from build123d import *

# Parameters (mm, degrees)
F0_W      = 108
F0_H      = 130
F1_DEPTH  = 70
F2_R      = 6.5
F3_DEPTH  = 70.001
F4_W      = 70
F4_H      = 50
F5_DEPTH  = 25
F6_W      = 108
F6_H      = 82
F7_DEPTH  = 25
F9_DEPTH  = 108.001
F10_R     = 10
F11_DEPTH = 20
F12_R     = 10
F13_DEPTH = 20
F14_W     = 44
F14_H     = 20
F14_W_2   = 20
F14_H_2   = 55
F15_DEPTH = 5


with BuildPart() as f1:
    # F0 (on Right) → F1 (new body)
    with BuildSketch(Plane.YZ):
        Rectangle(F0_W, F0_H)
    extrude(amount=-F1_DEPTH)

    # F2 (on face) → F3 (cut, through all)
    with BuildSketch(Plane(origin=(-70, 0, 0), x_dir=(0, -1, 0), z_dir=(-1, 0, 0))):
        with Locations((-42, 47)):
            Circle(F2_R)
        with Locations((42, 47)):
            Circle(F2_R)
        with Locations((-42, -47)):
            Circle(F2_R)
        with Locations((42, -47)):
            Circle(F2_R)
    extrude(amount=-F3_DEPTH, mode=Mode.SUBTRACT)

    # F4 (on face) → F5 (cut)
    with BuildSketch(Plane(origin=(0, 0, -65), x_dir=(1, 0, 0), z_dir=(0, 0, -1))):
        with Locations((-35, 0)):
            Rectangle(F4_W, F4_H)
    extrude(amount=-F5_DEPTH, mode=Mode.SUBTRACT)

    # F6 (on face) → F7 (cut)
    with BuildSketch(Plane(origin=(-70, 0, 0), x_dir=(0, -1, 0), z_dir=(-1, 0, 0))):
        with Locations((0, 24)):
            Rectangle(F6_W, F6_H)
    extrude(amount=-F7_DEPTH, mode=Mode.SUBTRACT)

    # F8 (on face) → F9 (cut, through all)
    with BuildSketch(Plane.XZ.offset(54)):
        Polygon((-65, -35), (-65, -17), (-70, -17), (-70, -40), align=None)
    extrude(amount=-F9_DEPTH, mode=Mode.SUBTRACT)

    # F10 (on face) → F11 (cut)
    with BuildSketch(Plane(origin=(-70, 0, 0), x_dir=(0, -1, 0), z_dir=(-1, 0, 0))):
        with Locations((-42, -47)):
            Circle(F10_R)
        with Locations((42, -47)):
            Circle(F10_R)
    extrude(amount=-F11_DEPTH, mode=Mode.SUBTRACT)

    # F12 (on face) → F13 (cut)
    with BuildSketch(Plane(origin=(-45, 0, 0), x_dir=(0, -1, 0), z_dir=(-1, 0, 0))):
        with Locations((-42, 47)):
            Circle(F12_R)
        with Locations((42, 47)):
            Circle(F12_R)
    extrude(amount=-F13_DEPTH, mode=Mode.SUBTRACT)

    # F14 (on face) → F15 (cut)
    with BuildSketch(Plane.YZ):
        with Locations((32, 0)):
            Rectangle(F14_W, F14_H)
        Rectangle(F14_W_2, F14_H)
        with Locations((0, 37.5)):
            Rectangle(F14_W_2, F14_H_2)
        with Locations((-32, 0)):
            Rectangle(F14_W, F14_H)
        with Locations((0, -37.5)):
            Rectangle(F14_W_2, F14_H_2)
    extrude(amount=-F15_DEPTH, mode=Mode.SUBTRACT)


solid = f1.part
Here's how the part is built. I have some questions about the finished solid (model axes, mm). A direction names the side the tool comes from. Coordinates: 2 decimals unless noted, no trailing zeros. Write each loop counter-clockwise with the first axis right and the second up, starting at its lowest first coordinate (ties: lowest second). Pieces come first, ordered by that corner, then holes.
Item 1: On a 3-axis mill with a long thin cutter (end or side, diameter ignored), from which of +Z, -Z, +X, -X, +Y, -Y can I reach the whole of each face in a straight line? I mean faces 1 (the flat face through (-35, -25, -53)), 2 (the flat face through (-65, -1, -26)), 3 (the flat face through (-2, 10, -25)), 4 (the cylindrical face through (-60.14, 44.17, -56.76)), 5 (the flat face through (-2, 32, -10)). Say none if no direction works.
Item 2: I want a section at A-A on z = 47. Write out the boundary of the cut face in (x, y).
Item 3: I want a section at B-B on y = 42. Write out the boundary of the cut face in (x, z), and give its area (3 significant figures).
Item 4: If I drill on line 1 (Y direction, x = -63, z = -47); line 2 (Z direction, x = -34, y = 42); line 3 (Y direction, x = -32.5, z = -51), over which ranges is the centre line in solid material (lowest first)?
Item 5: If we mould it in two halves opening along Z, with no side actions, what happens to faces 6 (the flat face through (-50, 42, -54)), 7 (the flat face through (-22, -1, 65)), 8 (the flat face through (-35, 25, -53))? For each: +Z half, -Z half, draft (parallel to the pull), parting line (faces both ways), or undercut.
Item 6: I want a section at D-D on z = -47. Write out the boundary of the cut face in (x, y), and give its area (3 significant figures).
Item 7: I want a section at C-C on x = -42. Write out the boundary of the cut face in (y, z).
Item 8: Will these pins go through, and if not, where does the flat tip stop? pin 1 (10 mm diameter, centred on y = -46, z = 45, fed in from -X); pin 2 (9 mm diameter, centred on y = -21, z = -27.5, fed in from -X); pin 3 (4 mm diameter, centred on x = -3.5, y = 22.5, fed in from -Z).
Findings below:
1. face 1: -Z, +X, -X
1. face 2: +Z, -X, +Y, -Y
1. face 3: +Z, -Z, +X
1. face 4: -X
1. face 5: +X, +Y, -Y
2. outline: (-45, -54) - (0, -54) - (0, -48.5) - (-25, -48.5) - (-25, -52) - (-45, -52) - close; (-45, -32) - (-25, -32) - (-25, -35.5) - (0, -35.5) - (0, -10) - (-5, -10) - (-5, 10) - (0, 10) - (0, 35.5) - (-25, 35.5) - (-25, 32) - (-45, 32) - close; (-45, 52) - (-25, 52) - (-25, 48.5) - (0, 48.5) - (0, 54) - (-45, 54) - close
3. outline: (-70, -65) - (0, -65) - (0, -53.5) - (-50, -53.5) - (-50, -57) - (-70, -57) - close; (-67, -37) - (-50, -37) - (-50, -40.5) - (0, -40.5) - (0, -10) - (-5, -10) - (-5, 10) - (0, 10) - (0, 40.5) - (-25, 40.5) - (-25, 37) - (-45, 37) - (-45, -17) - (-65, -17) - (-65, -35) - close; (-45, 57) - (-25, 57) - (-25, 53.5) - (0, 53.5) - (0, 65) - (-45, 65) - close
3. area: 5,080 mm2
4. line 1: y = -54 to -52, -32 to -25, 25 to 32, 52 to 54
4. line 2: z = -65 to -53.5, -40.5 to 37, 57 to 65
4. line 3: y = -54 to -47.12, -36.88 to -25, 25 to 36.88, 47.12 to 54
5. face 6: undercut
5. face 7: +Z half
5. face 8: draft
6. outline: (-70, -54) - (0, -54) - (0, -48.5) - (-50, -48.5) - (-50, -52) - (-70, -52) - close; (-70, -32) - (-50, -32) - (-50, -35.5) - (0, -35.5) - (0, -25) - (-70, -25) - close; (-70, 25) - (0, 25) - (0, 35.5) - (-50, 35.5) - (-50, 32) - (-70, 32) - close; (-70, 52) - (-50, 52) - (-50, 48.5) - (0, 48.5) - (0, 54) - (-70, 54) - close
6. area: 1,960 mm2
7. outline: (-54, -65) - (-25, -65) - (-25, -40) - (25, -40) - (25, -65) - (54, -65) - (54, 65) - (-54, 65) - close; hole circle Ø20 at (-42, 47); hole circle Ø13 at (-42, -47); hole circle Ø20 at (42, 47); hole circle Ø13 at (42, -47)
8. pin 1: stops at x = -25
8. pin 2: stops at x = -65
8. pin 3: stops at z = -40
